Geometry: final body of the model. Coordinates: model frame, mm. A direction names the side the tool comes from. Give positions to 0.01 mm unless a question says otherwise; leave off trailing zeros. Loops run counter-clockwise (first coordinate to the right, second up) from the corner with the lowest first, then second, coordinate; pieces in that order, holes last. Notation, with made-up numbers: M -16.5,3.5 L 4.5,3.5 A13 ccw 4.5,13.5 Z; hole C 21.5,52 d3. An arc over 180 degrees is marked long. One line per question, with ' | ' between items. Start each with the question number.
from build123d import *

# Parameters (mm, degrees)
BOSS_EXTRUDE2_DEPTH     = 15
CUT_EXTRUDE5_DEPTH      = 11
CUT_EXTRUDE5_DEPTH_BACK = 2


with BuildPart() as part:
    # Sketch3 → Boss-Extrude2 (new body)
    with BuildSketch(Plane(origin=(0, 0, 0), x_dir=(0, 0, -1), z_dir=(1, 0, 0))):
        Polygon((0, 0), (25.980762114, 15), (35, 15), (35, 11.334877204), (20.383272678, 4.827090915), (21.196745964, 3), (35, 9.145604647), (35, 0), align=None)
    extrude(amount=BOSS_EXTRUDE2_DEPTH)

    # Sketch7 → Cut-Extrude5 (cut, two sides)
    with BuildSketch(Plane(origin=(0, -5.37243013, -2.391960004), x_dir=(1, 0, 0), z_dir=(0, 0.913545458, 0.406736643))) as cut_extrude5_sk:
        with BuildLine():
            ThreePointArc((9.5, 25.075140664), (8.914213562, 26.489354226), (7.5, 27.075140664))
            Line((7.5, 27.075140664), (7.5, 23.075140664))
            ThreePointArc((7.5, 23.075140664), (8.914213562, 23.660927101), (9.5, 25.075140664))
        make_face()
        with BuildLine():
            Line((7.5, 23.075140664), (7.5, 27.075140664))
            ThreePointArc((7.5, 27.075140664), (5.5, 25.075140664), (7.5, 23.075140664))
        make_face()
    extrude(amount=CUT_EXTRUDE5_DEPTH, mode=Mode.SUBTRACT)
    extrude(cut_extrude5_sk.sketch, amount=-CUT_EXTRUDE5_DEPTH_BACK, mode=Mode.SUBTRACT)


solid = part.part
Q1. Section B-B, the plane z = -30. Output: boundary loops of the cut face in (x, y), plus the area to 3 significant figures.
Q2. Material intervals for L1, parallel to Y at x = 1.75, z = -13; L2, parallel to Y at x = 2, z = -32; L3, parallel to Z at x = 14.75, y = 8.75, sorted ascending.
Q3. Section C-C, the plane x = 10. Output: boundary loops of the cut face in (y, z).
Q4. Set-up query: faces 1 (the flat face through (7.395, 3.926, -20.784)), 2 (the flat face through (0, 6, -22)). Return all of +Z, -Z, +X, -X, +Y, -Y with unobstructed straight access to the full face (end or side cutting, diameter ignored); none if empty.
Q5. Contact query for flat-ended pins moving along their axis: pin 1 (4 mm diameter, centred on y = 6.5, z = -4, fed in from -X); pin 2 (8 mm diameter, centred on x = 6, z = -9, fed in from +Y); pin 3 (1 mm diameter, centred on x = 2.5, y = 6, fed in from +Z). Output: stop coordinate, or through.
Q6. Section A-A, the plane x = 8. Output: boundary loops of the cut face in (y, z).
Q7. Section D-D, the plane y = 1. Output: boundary loops of the cut face in (x, z), plus the area to 3 significant figures.
Q8. Draft query along Z for faces 3 (the flat face through (7.395, 7.395, -12.809)), 4 (the flat face through (7, 13, -35)), 5 (the flat face through (7.47, 3.01, -26.14)). Return one class per face: released by +Z, released by -Z, zero draft, split by the parting line, or undercut.
Model answer:
1) outline: M 0,0 L 15,0 L 15,6.92 L 0,6.92 Z; M 0,9.11 L 15,9.11 L 15,15 L 0,15 Z | area: 192 mm^2
2) L1: y = 0 to 7.51 | L2: y = 0 to 7.81, 10 to 15 | L3: z = -35 to -34.11, -29.19 to -15.16
3) outline: M 0,-35 L 9.15,-35 L 3,-21.2 L 4.83,-20.38 L 11.33,-35 L 15,-35 L 15,-25.98 L 0,0 Z
4) face 1: +X, -X | face 2: +Z, -Z, -X, +Y, -Y
5) pin 1: passes through | pin 2: stops at y = 7.51 | pin 3: stops at z = -9.53
6) outline: M 0,-35 L 9.15,-35 L 5.61,-27.07 L 3.79,-27.88 L 2.21,-24.34 L 4.04,-23.53 L 3,-21.2 L 4.83,-20.38 L 5.87,-22.72 L 11.63,-20.15 L 0,0 Z; M 7.44,-26.25 L 11.33,-35 L 15,-35 L 15,-25.98 L 13.58,-23.52 Z
7) outline: M 0,-35 L 15,-35 L 15,-1.73 L 0,-1.73 Z | area: 499 mm^2
8) face 3: released by +Z | face 4: released by -Z | face 5: undercut
